Source: CAD feature listing. Evaluate the final solid. Frame: model axes, mm. A direction names the side the tool comes from. Round coordinates to 2 decimals unless told otherwise and drop trailing zeros. Write each loop counter-clockwise with the first axis right and the second up, starting at its lowest first coordinate (ties: lowest second). Pieces come first, ordered by that corner, then holes. Notation, with made-up numbers: (69, 76) -> (97, 76) arc R12 cw to (97, 85) -> close; hole circle Ø2 at (63.25, 35.5). An arc over 180 degrees is marked (long way). Put each result on its own line as item: value.
```python
from build123d import *

# Parameters (mm, degrees)
BOSS_EXTRUDE1_DEPTH = 2
BOSS_EXTRUDE2_DEPTH = 8
SKETCH24_R          = 3.9
BOSS_EXTRUDE5_DEPTH = 4.4
SKETCH30_W          = 4.40861202
SKETCH30_H          = 1.324178481
CUT_EXTRUDE12_DEPTH = 16
CUT_EXTRUDE11_DEPTH = 23.928148639
FILLET1_R           = 1.5
SKETCH34_W          = 1.5
SKETCH34_H          = 1.5
CUT_EXTRUDE13_DEPTH = 8
SKETCH36_R          = 0.95
CUT_EXTRUDE15_DEPTH = 8
SKETCH37_R          = 2
CUT_EXTRUDE16_DEPTH = 4.5
SKETCH38_W          = 3
SKETCH38_H          = 1.25
CUT_EXTRUDE17_DEPTH = 3.6


with BuildPart() as part:
    # Sketch2 → Boss-Extrude1 (new body)
    with BuildSketch(Plane.XY):
        with BuildLine():
            Line((-2.5, 7.5), (-16.7, 7.5))
            Line((-16.7, 7.5), (-20.7, 3.793442666))
            Line((-20.7, 3.793442666), (-20.7, -4.031648778))
            Line((-20.7, -4.031648778), (-15.7, -7.5))
            Line((-15.7, -7.5), (-6.7, -7.5))
            Line((-6.7, -7.5), (-4.2, -5.6))
            ThreePointArc((-4.2, -5.6), (3.130495168, -6.260990337), (7, 0))
            ThreePointArc((7, 0), (4.949747468, 4.949747468), (0, 7))
            Line((0, 7), (0, 7.5))
            Line((0, 7.5), (-2.5, 7.5))
        make_face()
    extrude(amount=BOSS_EXTRUDE1_DEPTH)

    # Sketch4 → Boss-Extrude2 (add)
    with BuildSketch(Plane.XY.offset(2)):
        Polygon((-15.7, -7.5), (-6.7, -7.5), (-6.759079174, -4.5), (-7.7, -4.5), (-7.7, 2), (-5.5, 2), (-5.5, 5.3), (-2.5, 5.3), (-2.5, 7.5), (-16.7, 7.5), (-20.7, 3.793442666), (-20.7, -4.031648778), align=None)
    extrude(amount=BOSS_EXTRUDE2_DEPTH)

    # Sketch24 → Boss-Extrude5 (add)
    with BuildSketch(Plane.XY.offset(2)):
        Circle(SKETCH24_R)
    extrude(amount=BOSS_EXTRUDE5_DEPTH)

    # Sketch30 → Cut-Extrude12 (cut)
    with BuildSketch(Plane(origin=(-5.5, 0, 0), x_dir=(0, 0, -1), z_dir=(1, 0, 0))):
        with Locations((-4.20430601, 4.63791076)):
            Rectangle(SKETCH30_W, SKETCH30_H)
    extrude(amount=-CUT_EXTRUDE12_DEPTH, mode=Mode.SUBTRACT)

    # Sketch28 → Cut-Extrude11 (cut, through all)
    with BuildSketch(Plane.XY.offset(6.4)):
        with BuildLine():
            Line((-1, 0.979795897), (-1, -0.979795897))
            ThreePointArc((-1, -0.979795897), (1.4, 0), (-1, 0.979795897))
        make_face()
    extrude(amount=-CUT_EXTRUDE11_DEPTH, mode=Mode.SUBTRACT)

    # Fillet1
    # the kernel refuses this fillet: 1.5 mm, written as the material it takes off along each edge
    with BuildSketch(Plane(origin=(-15.230677435, -6, 1.5), x_dir=(-0.5699665637840448, -0.8216678867816415, 0), z_dir=(0, 0, -1))) as fillet1_piece_1_section:
        Polygon((0, 0), (FILLET1_R * 1.02, 0), (FILLET1_R * 1.02, -FILLET1_R * 0.319139344377), (FILLET1_R * 0.838101244517, -FILLET1_R * 0.58136589506), align=None)
    fillet1_piece_1 = extrude(amount=FILLET1_R * 1.02, mode=Mode.PRIVATE)
    fillet1_piece_1 = fillet1_piece_1 - Plane(origin=(-15.230677435, -6, 1.5), x_dir=(0.29860685961507855, 0.9543762064253388, 0), z_dir=(0, 0, -1)) * Sphere(FILLET1_R, mode=Mode.PRIVATE)
    add(fillet1_piece_1, mode=Mode.SUBTRACT)
    with BuildSketch(Plane(origin=(-16.11186344, 6, 1.5), x_dir=(-0.6796897201843015, 0.7334997506991983, 0), z_dir=(0, 0, -1))) as fillet1_piece_2_section:
        Polygon((0, 0), (FILLET1_R * 1.02, 0), (FILLET1_R * 1.02, FILLET1_R * 0.399932860855), (FILLET1_R * 0.748169745713, FILLET1_R * 0.693283514588), align=None)
    fillet1_piece_2 = extrude(amount=FILLET1_R * 1.02, mode=Mode.PRIVATE)
    fillet1_piece_2 = fillet1_piece_2 - Plane(origin=(-16.11186344, 6, 1.5), x_dir=(0.3650344157067945, -0.9309940254102596, 0), z_dir=(0, 0, -1)) * Sphere(FILLET1_R, mode=Mode.PRIVATE)
    add(fillet1_piece_2, mode=Mode.SUBTRACT)
    with BuildSketch(Plane(origin=(-19.2, 3.138411196, 1.5), x_dir=(-0.6796897201843015, 0.7334997506991983, 0), z_dir=(0, 0, -1))) as fillet1_piece_3_section:
        Polygon((0, 0), (FILLET1_R * 1.02, 0), (FILLET1_R * 1.02, -FILLET1_R * 0.445421399395), (FILLET1_R * 0.693283514588, -FILLET1_R * 0.748169745713), align=None)
    fillet1_piece_3 = extrude(amount=FILLET1_R * 1.02, mode=Mode.PRIVATE)
    fillet1_piece_3 = fillet1_piece_3 - Plane(origin=(-19.2, 3.138411196, 1.5), x_dir=(0.9164304993244992, -0.40019387789901173, 0), z_dir=(0, 0, -1)) * Sphere(FILLET1_R, mode=Mode.PRIVATE)
    add(fillet1_piece_3, mode=Mode.SUBTRACT)
    with BuildSketch(Plane(origin=(-19.2, -3.246599046, 1.5), x_dir=(-0.5699665637840448, -0.8216678867816415, 0), z_dir=(0, 0, -1))) as fillet1_piece_4_section:
        Polygon((0, 0), (FILLET1_R * 1.02, 0), (FILLET1_R * 1.02, FILLET1_R * 0.533833817771), (FILLET1_R * 0.58136589506, FILLET1_R * 0.838101244517), align=None)
    fillet1_piece_4 = extrude(amount=FILLET1_R * 1.02, mode=Mode.PRIVATE)
    fillet1_piece_4 = fillet1_piece_4 - Plane(origin=(-19.2, -3.246599046, 1.5), x_dir=(0.8859928227090906, 0.46369895202380795, 0), z_dir=(0, 0, -1)) * Sphere(FILLET1_R, mode=Mode.PRIVATE)
    add(fillet1_piece_4, mode=Mode.SUBTRACT)
    with BuildSketch(Plane(origin=(-15.230677435, -7.5, 0), x_dir=(0, 1, 0), z_dir=(1, 0, 0))) as fillet1_piece_5_section:
        with BuildLine():
            CenterArc((FILLET1_R, FILLET1_R), FILLET1_R, 180, 90)
            Line((0, FILLET1_R), (0, 0))
            Line((0, 0), (FILLET1_R, 0))
        make_face()
    fillet1_piece_5 = extrude(amount=12.280677435, mode=Mode.PRIVATE)
    fillet1_piece_5 = split(fillet1_piece_5, bisect_by=Plane(origin=(-9.092127217, -9.318016685, 0.3282266), z_dir=(-0.6050832675335577, 0.7961621941231027, 0)), keep=Keep.TOP, mode=Mode.PRIVATE)
    add(fillet1_piece_5, mode=Mode.SUBTRACT)
    with BuildSketch(Plane(origin=(3.75, 7.5, 0), x_dir=(0, 0, 1), z_dir=(-1, 0, 0))) as fillet1_piece_6:
        with BuildLine():
            CenterArc((FILLET1_R, -FILLET1_R), FILLET1_R, 90, 90)
            Line((0, -FILLET1_R), (0, 0))
            Line((0, 0), (FILLET1_R, 0))
        make_face()
    extrude(amount=19.86186344, mode=Mode.SUBTRACT)
    with BuildSketch(Plane(origin=(-17.13139802, 7.100249626, 0), x_dir=(0.6796897201843014, -0.7334997506991981, 0), z_dir=(-0.7334997506991983, -0.6796897201843015, 0))) as fillet1_piece_7:
        with BuildLine():
            CenterArc((FILLET1_R, FILLET1_R), FILLET1_R, 180, 90)
            Line((0, FILLET1_R), (0, 0))
            Line((0, 0), (FILLET1_R, 0))
        make_face()
    extrude(amount=4.21013989, mode=Mode.SUBTRACT)
    with BuildSketch(Plane(origin=(-20.054949846, -4.479100876, 0), x_dir=(0.5699665637840448, 0.8216678867816416, 0), z_dir=(0.8216678867816415, -0.5699665637840448, 0))) as fillet1_piece_8:
        with BuildLine():
            CenterArc((FILLET1_R, FILLET1_R), FILLET1_R, 180, 90)
            Line((0, FILLET1_R), (0, 0))
            Line((0, 0), (FILLET1_R, 0))
        make_face()
    extrude(amount=4.830811364, mode=Mode.SUBTRACT)
    with BuildSketch(Plane(origin=(-20.7, 3.138411196, 0), x_dir=(1, 0, 0), z_dir=(0, -1, 0))) as fillet1_piece_9:
        with BuildLine():
            CenterArc((FILLET1_R, FILLET1_R), FILLET1_R, 180, 90)
            Line((0, FILLET1_R), (0, 0))
            Line((0, 0), (FILLET1_R, 0))
        make_face()
    extrude(amount=6.385010242, mode=Mode.SUBTRACT)
    with BuildSketch(Plane(origin=(-15.7, -7.5, 1.5), x_dir=(1, 0, 0), z_dir=(0, 0, 1))) as fillet1_piece_10:
        with BuildLine():
            CenterArc((FILLET1_R * 0.312881710173, FILLET1_R), FILLET1_R, 235.252105822, 34.747894178)
            Line((-FILLET1_R * 0.257084853611, FILLET1_R * 0.178332113218), (0, 0))
            Line((0, 0), (FILLET1_R * 0.312881710173, 0))
        make_face()
    extrude(amount=9.673306413, mode=Mode.SUBTRACT)
    with BuildSketch(Plane(origin=(-20.7, -4.031648778, 1.5), x_dir=(0, 1, 0), z_dir=(0, 0, 1))) as fillet1_piece_11:
        with BuildLine():
            CenterArc((FILLET1_R * 0.523366488011, -FILLET1_R), FILLET1_R, 90, 55.252105822)
            Line((-FILLET1_R * 0.298301398771, -FILLET1_R * 0.430033436216), (0, 0))
            Line((0, 0), (FILLET1_R * 0.523366488011, 0))
        make_face()
    extrude(amount=10.46262433, mode=Mode.SUBTRACT)
    with BuildSketch(Plane(origin=(-20.7, 3.793442666, 1.5), x_dir=(0.7334997506991984, 0.6796897201843014, 0), z_dir=(0, 0, 1))) as fillet1_piece_12:
        with BuildLine():
            CenterArc((FILLET1_R * 0.436687646465, -FILLET1_R), FILLET1_R, 90, 47.18059856)
            Line((-FILLET1_R * 0.296812104234, -FILLET1_R * 0.320310279816), (0, 0))
            Line((0, 0), (FILLET1_R * 0.436687646465, 0))
        make_face()
    extrude(amount=10.137578674, mode=Mode.SUBTRACT)
    with BuildSketch(Plane(origin=(-16.7, 7.5, 1.5), x_dir=(1, 0, 0), z_dir=(0, 0, 1))) as fillet1_piece_13:
        with BuildLine():
            CenterArc((FILLET1_R * 0.392091040054, -FILLET1_R), FILLET1_R, 90, 42.81940144)
            Line((-FILLET1_R * 0.287598680131, -FILLET1_R * 0.266500249301), (0, 0))
            Line((0, 0), (FILLET1_R * 0.392091040054, 0))
        make_face()
    extrude(amount=9.9703414, mode=Mode.SUBTRACT)

    # Sketch34 → Cut-Extrude13 (cut, along a direction that is not the sketch's normal)
    with BuildSketch(Plane.XZ.offset(-2)):
        with Locations((-6.95, 10)):
            Rectangle(SKETCH34_W, SKETCH34_H)
    extrude(amount=-CUT_EXTRUDE13_DEPTH, dir=(0.6685833876565112, -0.7436371788377336, 0), mode=Mode.SUBTRACT)

    # Sketch36 → Cut-Extrude15 (cut)
    with BuildSketch(Plane.XY.offset(10)):
        with Locations((-11.7, 0)):
            Circle(SKETCH36_R)
        with Locations((-16.7, 0)):
            Circle(SKETCH36_R)
    extrude(amount=-CUT_EXTRUDE15_DEPTH, mode=Mode.SUBTRACT)

    # Sketch37 → Cut-Extrude16 (cut)
    with BuildSketch(Plane(origin=(0, 0, 0), x_dir=(-1, 0, 0), z_dir=(0, 0, -1))):
        with Locations((11.7, 0)):
            Circle(SKETCH37_R)
        with Locations((16.7, 0)):
            Circle(SKETCH37_R)
    extrude(amount=-CUT_EXTRUDE16_DEPTH, mode=Mode.SUBTRACT)

    # Sketch38 → Cut-Extrude17 (cut)
    with BuildSketch(Plane.XY.offset(10)):
        with Locations((-4, 5.925)):
            Rectangle(SKETCH38_W, SKETCH38_H)
    extrude(amount=-CUT_EXTRUDE17_DEPTH, mode=Mode.SUBTRACT)


with BuildPart() as body_2:
    # Split1: the piece on the far side of the plane
    add(part.part)
    split(bisect_by=Plane.XY.offset(6.4), keep=Keep.BOTTOM)


with BuildPart() as part_1:
    add(part.part)

    # Split1
    split(bisect_by=Plane.XY.offset(6.4), keep=Keep.TOP)


solid = part_1.part
```
Q1. Cut plane A-A on y = 0. Output: boundary loops of the cut face in (x, z).
Ans:
outline: (-20.7, 6.4) -> (-17.65, 6.4) -> (-17.65, 10) -> (-20.7, 10) -> close; (-15.75, 6.4) -> (-12.65, 6.4) -> (-12.65, 10) -> (-15.75, 10) -> close; (-10.75, 6.4) -> (-7.7, 6.4) -> (-7.7, 10) -> (-10.75, 10) -> close
Q2. Cut plane B-B on z = 7.5. Output: boundary loops of the cut face in (x, y).
Ans:
outline: (-20.7, -3.25) arc R1.5 ccw to (-20.05, -4.48) -> (-16.09, -7.23) arc R1.5 ccw to (-15.23, -7.5) -> (-6.7, -7.5) -> (-6.76, -4.5) -> (-7.7, -4.5) -> (-7.7, 2) -> (-5.5, 2) -> (-5.5, 6.55) -> (-2.5, 6.55) -> (-2.5, 7.5) -> (-16.11, 7.5) arc R1.5 ccw to (-17.13, 7.1) -> (-20.22, 4.24) arc R1.5 ccw to (-20.7, 3.14) -> close; hole circle Ø1.9 at (-16.7, 0); hole circle Ø1.9 at (-11.7, 0)
Q3. Cut plane D-D on y = 5. Output: boundary loops of the cut face in (x, z), and give its area (3 significant figures).
Ans:
outline: (-19.4, 6.41) -> (-5.5, 6.41) -> (-5.5, 10) -> (-8.9, 10) -> (-8.9, 9.25) -> (-10.4, 9.25) -> (-10.4, 10) -> (-19.4, 10) -> close
area: 48.8 mm^2
Q4. Reachability of faces 4 (the flat face through (-4, 6.55, 8)), 5 (the flat face through (-9.4, 4.7, 9.25)), 6 (the cylindrical face through (-20.534, -3.933, 8.175)) from +Z, -Z, +X, -X, +Y, -Y: full face, straight path, thin tool, end or side. Return the list, or none.
Ans:
face 4: +Z, -Z, +X, -Y
face 5: +Z
face 6: +Z, -Z, -X, -Y
Q5. Material intervals for line 1 (Y direction, x = -5.25, z = 7.8); line 2 (X direction, y = 2.25, z = 7.9); line 3 (Y direction, x = -16.75, z = 8.15), sorted ascending. Write a range as [from, to].
Ans:
line 1: y = [6.55, 7.5]
line 2: x = [-20.7, -5.5]
line 3: y = [-6.77, -0.95], [0.95, 7.36]
Q6. Pin query (flat end, axial travel): pin 1 (1.8 mm diameter, centred on y = 5.5, z = 8.5, fed in from +X); pin 2 (1.5 mm diameter, centred on y = -2.5, z = 8.5, fed in from +X); pin 3 (1.1 mm diameter, centred on x = -16.7, y = 0, fed in from -Z); pin 4 (2 mm diameter, centred on x = -18, z = 8.5, fed in from -Y). Return the tip coordinate at first contact, or that it passes through.
Ans:
pin 1: stops at x = -5.5
pin 2: stops at x = -7.7
pin 3: passes through
pin 4: stops at y = -6.6
Q7. Draft query along X for faces 1 (the flat face through (-10.138, 4.712, 9.62)), 2 (the flat face through (-18.098, -5.837, 8.175)), 3 (the flat face through (-7, 2, 8)). Return one class per face: +X half, -X half, draft (parallel to the pull), parting line (faces both ways), or undercut.
Ans:
face 1: undercut
face 2: -X half
face 3: draft
